Read the model definition and answer for the solid it produces. Units are mm, in the model's axes. Give positions to 0.01 mm unless a question says otherwise; leave off trailing zeros. Loops run counter-clockwise (first coordinate to the right, second up) from the corner with the lowest first, then second, coordinate; pieces in that order, holes last. Notation, with made-up numbers: (22, 50) - (30, 50) arc R8 ccw to (30, 64) - close; hole circle Ø2 at (40.5, 28). An arc over 180 degrees is marked (long way). Put each result on its own line as item: value. Start each with the question number.
1. A cutting plane is placed at B-B, the plane y = -1.65. Determine the outline of the cut face in (x, z).
2. A cutting plane is placed at D-D, the plane z = 1. Determine the outline of the cut face in (x, y).
3. A cutting plane is placed at C-C, the plane z = -3.5. Determine the outline of the cut face in (x, y), plus the area to 3 significant figures.
4. A cutting plane is placed at A-A, the plane z = -1.5. Determine the outline of the cut face in (x, y), plus the area to 3 significant figures.
5. Consider L1, parallel to X at y = -1.75, z = -1; L2, parallel to X at y = -1, z = -2.5; L3, parallel to X at y = -1.75, z = 2. Determine where each line is inside the solid, lowest interval first. Write a range as from..to.
```python
from build123d import *

# Parameters (mm, degrees)
BOSS_EXTRUDE1_DEPTH = 2


with BuildPart() as part:
    # Sketch1 → Boss-Extrude1 (new body)
    with BuildSketch(Plane(origin=(0, 0, 0), x_dir=(1, 0, 0), z_dir=(0, 1, 0))):
        with BuildLine():
            ThreePointArc((-9.493876204, 2.669468268), (-8.362505354, 2.200839118), (-7.893876204, 1.069468268))
            Line((-7.893876204, 1.069468268), (-4.893876204, 1.069468268))
            ThreePointArc((-4.893876204, 1.069468268), (-6.24118501, 4.322159461), (-9.493876204, 5.669468268))
            Line((-9.493876204, 5.669468268), (-9.493876204, 2.669468268))
        make_face()
        with BuildLine():
            ThreePointArc((-9.493876204, -0.530531732), (-11.093876204, 1.069468268), (-9.493876204, 2.669468268))
            Line((-9.493876204, 2.669468268), (-9.493876204, 5.669468268))
            ThreePointArc((-9.493876204, 5.669468268), (-14.093876204, 1.069468268), (-9.493876204, -3.530531732))
            Line((-9.493876204, -3.530531732), (-9.493876204, -0.530531732))
        make_face()
        with BuildLine():
            Line((-4.893876204, 1.069468268), (-7.893876204, 1.069468268))
            ThreePointArc((-7.893876204, 1.069468268), (-8.362505354, -0.061902582), (-9.493876204, -0.530531732))
            Line((-9.493876204, -0.530531732), (-9.493876204, -3.530531732))
            ThreePointArc((-9.493876204, -3.530531732), (-6.24118501, -2.183222925), (-4.893876204, 1.069468268))
        make_face()
        with BuildLine():
            Line((26.016123796, 1.069468268), (-4.893876204, 1.069468268))
            ThreePointArc((-4.893876204, 1.069468268), (-6.24118501, -2.183222925), (-9.493876204, -3.530531732))
            Line((-9.493876204, -3.530531732), (30.616123796, -3.530531732))
            ThreePointArc((30.616123796, -3.530531732), (27.363432603, -2.183222925), (26.016123796, 1.069468268))
        make_face()
        with BuildLine():
            ThreePointArc((-9.493876204, 5.669468268), (-6.24118501, 4.322159461), (-4.893876204, 1.069468268))
            Line((-4.893876204, 1.069468268), (26.016123796, 1.069468268))
            ThreePointArc((26.016123796, 1.069468268), (27.363432603, 4.322159461), (30.616123796, 5.669468268))
            Line((30.616123796, 5.669468268), (-9.493876204, 5.669468268))
        make_face()
        with BuildLine():
            Line((29.016123796, 1.069468268), (26.016123796, 1.069468268))
            ThreePointArc((26.016123796, 1.069468268), (27.363432603, -2.183222925), (30.616123796, -3.530531732))
            Line((30.616123796, -3.530531732), (30.616123796, -0.530531732))
            ThreePointArc((30.616123796, -0.530531732), (29.484752947, -0.061902582), (29.016123796, 1.069468268))
        make_face()
        with BuildLine():
            ThreePointArc((30.616123796, 5.669468268), (27.363432603, 4.322159461), (26.016123796, 1.069468268))
            Line((26.016123796, 1.069468268), (29.016123796, 1.069468268))
            ThreePointArc((29.016123796, 1.069468268), (29.484752947, 2.200839118), (30.616123796, 2.669468268))
            Line((30.616123796, 2.669468268), (30.616123796, 5.669468268))
        make_face()
        with BuildLine():
            ThreePointArc((35.216123796, 1.069468268), (33.86881499, 4.322159461), (30.616123796, 5.669468268))
            Line((30.616123796, 5.669468268), (30.616123796, 2.669468268))
            ThreePointArc((30.616123796, 2.669468268), (31.747494646, 2.200839118), (32.216123796, 1.069468268))
            ThreePointArc((32.216123796, 1.069468268), (31.747494646, -0.061902582), (30.616123796, -0.530531732))
            Line((30.616123796, -0.530531732), (30.616123796, -3.530531732))
            ThreePointArc((30.616123796, -3.530531732), (33.86881499, -2.183222925), (35.216123796, 1.069468268))
        make_face()
    extrude(amount=-BOSS_EXTRUDE1_DEPTH)


solid = part.part
```
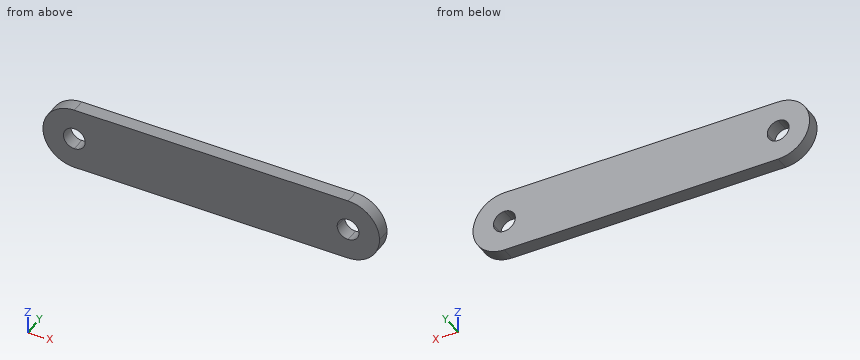
Return value:
1. outline: (-9.49, -5.67) - (30.62, -5.67) arc R4.6 ccw to (30.62, 3.53) - (-9.49, 3.53) arc R4.6 ccw to start; hole circle Ø3.2 at (-9.49, -1.07); hole circle Ø3.2 at (30.62, -1.07)
2. outline: (-13.6, -2) - (34.72, -2) - (34.72, 0) - (-13.6, 0) - close
3. outline: (-13.4, -2) - (34.52, -2) - (34.52, 0) - (-13.4, 0) - close
3. area: 95.8 mm2
4. outline: (-14.07, -2) - (-11.03, -2) - (-11.03, 0) - (-14.07, 0) - close; (-7.95, -2) - (29.08, -2) - (29.08, 0) - (-7.95, 0) - close; (32.16, -2) - (35.2, -2) - (35.2, 0) - (32.16, 0) - close
4. area: 86.2 mm2
5. L1: x = -14.09..-11.09, -7.9..29.02, 32.21..35.22
5. L2: x = -13.87..-10.21, -8.78..29.9, 31.33..34.99
5. L3: x = -12.92..34.04
